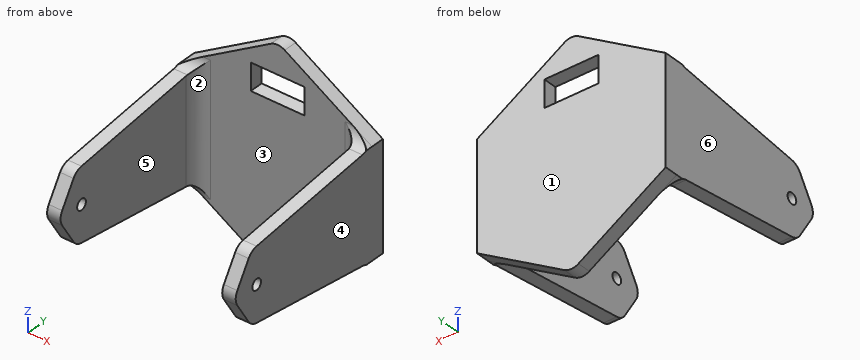
```python
from build123d import *

# Parameters (mm, degrees)
F0_W         = 5
F0_H         = 40
F1_DEPTH     = 70
F3_DEPTH     = 5
F4_R         = 2
F5_DEPTH     = 97.2
F7_DEPTH     = 83.6
F8_T4_DEPTH  = 65
F8_T10_DEPTH = 65
F8_T16_DEPTH = 5
F8_T21_DEPTH = 5
F8_T26_DEPTH = 5
F8_T31_DEPTH = 5
F8_T37_DEPTH = 16.0458347789
F8_T42_DEPTH = 65
F8_T50_DEPTH = 16.0458347789
F8_T55_DEPTH = 65
F8_T63_DEPTH = 16.0458347789
F8_T68_DEPTH = 65
F8_T76_DEPTH = 65
F8_T81_DEPTH = 16.0458347789
F8_T85_DEPTH = 20.294112478
F9_W         = 20
F9_H         = 10
F10_DEPTH    = 25


# Not quite as in the source:
# - a fillet or chamfer that OpenCascade refuses, or shapes differently, is made with other operations: its cross-section is extruded or revolved along the edge and cut away or added


with BuildPart() as f1:
    # F0 (on Front) → F1 (new body)
    with BuildSketch(Plane.XZ):
        with Locations((-32.5, 0)):
            Rectangle(F0_W, F0_H)
    extrude(amount=F1_DEPTH)



with BuildPart() as f1b:
    # F0 (on Front) → F1, piece 2 (new body)
    with BuildSketch(Plane.XZ):
        with Locations((32.5, 0)):
            Rectangle(F0_W, F0_H)
    extrude(amount=F1_DEPTH)


with BuildPart() as f1_1:
    add(f1.part)

    add(f1b.part)  # F3 merges F1b
    # F2 (on face) → F3 (join)
    with BuildSketch(Plane(origin=(0, 0, 0), x_dir=(-1, 0, 0), z_dir=(0, 1, 0))):
        Polygon((-35, -20), (0, -41.4117574692), (35, -20), (35, 20), (0, 41.4117574692), (-35, 20), align=None)
    extrude(amount=F3_DEPTH)

    # F4 (on face) → F5 (cut)
    with BuildSketch(Plane(origin=(-35, 0, 0), x_dir=(0, -1, 0), z_dir=(-1, 0, 0))):
        with Locations((52.9787652194, 0)):
            Circle(F4_R)
    extrude(amount=-F5_DEPTH, mode=Mode.SUBTRACT)

    # F6 (on face) → F7 (cut)
    with BuildSketch(Plane(origin=(-35, 0, 0), x_dir=(0, -1, 0), z_dir=(-1, 0, 0))):
        with BuildLine():
            Line((98.4306931496, 40.8057309687), (0, 20))
            Line((0, 20), (53.01884554, 13.4261534673))
            ThreePointArc((53.01884554, 13.4261534673), (55.107028482, 12.6702755654), (56.6618948527, 11.084636902))
            Line((56.6618948527, 11.084636902), (61.8706015463, 2.6204867239))
            ThreePointArc((61.8706015463, 2.6204867239), (62.6123097139, 0), (61.8706015463, -2.6204867239))
            Line((61.8706015463, -2.6204867239), (56.6618948527, -11.084636902))
            ThreePointArc((56.6618948527, -11.084636902), (55.107028482, -12.6702755654), (53.01884554, -13.4261534673))
            Line((53.01884554, -13.4261534673), (0, -20))
            Line((0, -20), (98.4306931496, -42.0177839696))
            Line((98.4306931496, -42.0177839696), (98.4306931496, 40.8057309687))
        make_face()
    extrude(amount=-F7_DEPTH, mode=Mode.SUBTRACT)

    # F8: fillet of radius 5 on 8 edges, made by hand


with BuildPart() as f8_tool2:
    # F8_s3 → F8_t4 (new body)
    with BuildSketch(Plane.XY.offset(32.5)):
        with BuildLine():
            ThreePointArc((25, 0), (28.5355339059, -1.4644660941), (30, -5))
            Line((30, -5), (30, 0))
            Line((30, 0), (25, 0))
        make_face()
    extrude(amount=-F8_T4_DEPTH)

    split(bisect_by=Plane(origin=(0, -2.4422683248, 19.6971813136), x_dir=(1, 0, 0), z_dir=(0, 0.1230485039, -0.9924006578)), keep=Keep.TOP)

    split(bisect_by=Plane(origin=(0, -2.4422683248, -19.6971813136), x_dir=(1, 0, 0), z_dir=(0, 0.1230485039, 0.9924006578)), keep=Keep.TOP)


with BuildPart() as f1_2:
    add(f1_1.part)

    # F8_t1: union F8_tool2
    add(f8_tool2.part)


with BuildPart() as f8_tool8:
    # F8_s9 → F8_t10 (new body)
    with BuildSketch(Plane.XY.offset(-32.5)):
        with BuildLine():
            ThreePointArc((-25, 0), (-28.5355339059, -1.4644660941), (-30, -5))
            Line((-30, -5), (-30, 0))
            Line((-30, 0), (-25, 0))
        make_face()
    extrude(amount=F8_T10_DEPTH)

    split(bisect_by=Plane(origin=(0, -2.4422683248, -19.6971813136), x_dir=(1, 0, 0), z_dir=(0, 0.1230485039, 0.9924006578)), keep=Keep.TOP)

    split(bisect_by=Plane(origin=(0, -2.4422683248, 19.6971813136), x_dir=(1, 0, 0), z_dir=(0, 0.1230485039, -0.9924006578)), keep=Keep.TOP)


with BuildPart() as f1_3:
    add(f1_2.part)

    # F8_t7: union F8_tool8
    add(f8_tool8.part)


with BuildPart() as f8_tool14:
    # F8_s15 → F8_t16 (new body)
    with BuildSketch(Plane.YZ.offset(35)):
        with BuildLine():
            ThreePointArc((-4.3847574804, 19.4563306223), (-1.2532539052, 21.1074588458), (0, 24.4183339115))
            Line((0, 24.4183339115), (0, 20))
            Line((0, 20), (-4.3847574804, 19.4563306223))
        make_face()
    extrude(amount=-F8_T16_DEPTH)

    split(bisect_by=Plane(origin=(18.4348816442, 0, 30.1339513338), x_dir=(0, 1, 0), z_dir=(-0.5218557601, 0, -0.8530337424)), keep=Keep.TOP)


with BuildPart() as f1_4:
    add(f1_3.part)

    # F8_t13: union F8_tool14
    add(f8_tool14.part)


with BuildPart() as f8_tool19:
    # F8_s20 → F8_t21 (new body)
    with BuildSketch(Plane.YZ.offset(-30)):
        with BuildLine():
            ThreePointArc((0, 24.4183339115), (-1.2532539052, 21.1074588458), (-4.3847574804, 19.4563306223))
            Line((-4.3847574804, 19.4563306223), (0, 20))
            Line((0, 20), (0, 24.4183339115))
        make_face()
    extrude(amount=-F8_T21_DEPTH)

    split(bisect_by=Plane(origin=(-18.4348816442, 0, 30.1339513338), x_dir=(0, 1, 0), z_dir=(0.5218557601, 0, -0.8530337424)), keep=Keep.TOP)


with BuildPart() as f1_5:
    add(f1_4.part)

    # F8_t18: union F8_tool19
    add(f8_tool19.part)


with BuildPart() as f8_tool24:
    # F8_s25 → F8_t26 (new body)
    with BuildSketch(Plane.YZ.offset(-35)):
        with BuildLine():
            ThreePointArc((0, -24.4183339115), (-1.2532539052, -21.1074588458), (-4.3847574804, -19.4563306223))
            Line((-4.3847574804, -19.4563306223), (0, -20))
            Line((0, -20), (0, -24.4183339115))
        make_face()
    extrude(amount=F8_T26_DEPTH)

    split(bisect_by=Plane(origin=(-18.4348816442, 0, -30.1339513338), x_dir=(0, 1, 0), z_dir=(0.5218557601, 0, 0.8530337424)), keep=Keep.TOP)


with BuildPart() as f1_6:
    add(f1_5.part)

    # F8_t23: union F8_tool24
    add(f8_tool24.part)


with BuildPart() as f8_tool29:
    # F8_s30 → F8_t31 (new body)
    with BuildSketch(Plane.YZ.offset(30)):
        with BuildLine():
            ThreePointArc((-4.3847574804, -19.4563306223), (-1.2532539052, -21.1074588458), (0, -24.4183339115))
            Line((0, -24.4183339115), (0, -20))
            Line((0, -20), (-4.3847574804, -19.4563306223))
        make_face()
    extrude(amount=F8_T31_DEPTH)

    split(bisect_by=Plane(origin=(18.4348816442, 0, -30.1339513338), x_dir=(0, 1, 0), z_dir=(-0.5218557601, 0, 0.8530337424)), keep=Keep.TOP)


with BuildPart() as f1_7:
    add(f1_6.part)

    # F8_t28: union F8_tool29
    add(f8_tool29.part)


with BuildPart() as f8_tool35:
    # F8_s36 → F8_t37 (new body)
    with BuildSketch(Plane.YZ.offset(35)):
        with BuildLine():
            ThreePointArc((-4.3847574804, 19.4563306223), (-1.2532539052, 21.1074588458), (0, 24.4183339115))
            Line((0, 24.4183339115), (0, 20))
            Line((0, 20), (-4.3847574804, 19.4563306223))
        make_face()
    extrude(amount=-F8_T37_DEPTH)

    split(bisect_by=Plane(origin=(18.4348816442, 0, 30.1339513338), x_dir=(0, 1, 0), z_dir=(-0.5218557601, 0, -0.8530337424)), keep=Keep.TOP)

    split(bisect_by=Plane.YZ.offset(30), keep=Keep.BOTTOM)


with BuildPart() as f8_tool40:
    # F8_s41 → F8_t42 (new body)
    with BuildSketch(Plane.XY.offset(32.5)):
        with BuildLine():
            ThreePointArc((25, 0), (28.5355339059, -1.4644660941), (30, -5))
            Line((30, -5), (30, 0))
            Line((30, 0), (25, 0))
        make_face()
    extrude(amount=-F8_T42_DEPTH)

    split(bisect_by=Plane(origin=(18.4348816442, 0, 30.1339513338), x_dir=(0, 1, 0), z_dir=(-0.5218557601, 0, -0.8530337424)), keep=Keep.TOP)

    split(bisect_by=Plane(origin=(0, -2.4422683248, 19.6971813136), x_dir=(1, 0, 0), z_dir=(0, -0.1230485039, 0.9924006578)), keep=Keep.TOP)


with BuildPart() as f8_tool35_1:
    add(f8_tool35.part)

    # F8_t45: intersect F8_tool40
    add(f8_tool40.part, mode=Mode.INTERSECT)


with BuildPart() as f1_8:
    add(f1_7.part)

    # F8_t33: union F8_tool35
    add(f8_tool35_1.part)


with BuildPart() as f8_tool48:
    # F8_s49 → F8_t50 (new body)
    with BuildSketch(Plane.YZ.offset(18.9541652211)):
        with BuildLine():
            ThreePointArc((-4.3847574804, -19.4563306223), (-1.2532539052, -21.1074588458), (0, -24.4183339115))
            Line((0, -24.4183339115), (0, -20))
            Line((0, -20), (-4.3847574804, -19.4563306223))
        make_face()
    extrude(amount=F8_T50_DEPTH)

    split(bisect_by=Plane(origin=(18.4348816442, 0, -30.1339513338), x_dir=(0, 1, 0), z_dir=(-0.5218557601, 0, 0.8530337424)), keep=Keep.TOP)

    split(bisect_by=Plane.YZ.offset(30), keep=Keep.BOTTOM)


with BuildPart() as f8_tool53:
    # F8_s54 → F8_t55 (new body)
    with BuildSketch(Plane.XY.offset(32.5)):
        with BuildLine():
            ThreePointArc((25, 0), (28.5355339059, -1.4644660941), (30, -5))
            Line((30, -5), (30, 0))
            Line((30, 0), (25, 0))
        make_face()
    extrude(amount=-F8_T55_DEPTH)

    split(bisect_by=Plane(origin=(18.4348816442, 0, -30.1339513338), x_dir=(0, 1, 0), z_dir=(-0.5218557601, 0, 0.8530337424)), keep=Keep.TOP)

    split(bisect_by=Plane(origin=(0, -2.4422683248, -19.6971813136), x_dir=(1, 0, 0), z_dir=(0, -0.1230485039, -0.9924006578)), keep=Keep.TOP)


with BuildPart() as f8_tool48_1:
    add(f8_tool48.part)

    # F8_t58: intersect F8_tool53
    add(f8_tool53.part, mode=Mode.INTERSECT)


with BuildPart() as f1_9:
    add(f1_8.part)

    # F8_t46: union F8_tool48
    add(f8_tool48_1.part)


with BuildPart() as f8_tool61:
    # F8_s62 → F8_t63 (new body)
    with BuildSketch(Plane.YZ.offset(-35)):
        with BuildLine():
            ThreePointArc((0, -24.4183339115), (-1.2532539052, -21.1074588458), (-4.3847574804, -19.4563306223))
            Line((-4.3847574804, -19.4563306223), (0, -20))
            Line((0, -20), (0, -24.4183339115))
        make_face()
    extrude(amount=F8_T63_DEPTH)

    split(bisect_by=Plane(origin=(-18.4348816442, 0, -30.1339513338), x_dir=(0, 1, 0), z_dir=(0.5218557601, 0, 0.8530337424)), keep=Keep.TOP)

    split(bisect_by=Plane.YZ.offset(-30), keep=Keep.TOP)


with BuildPart() as f8_tool66:
    # F8_s67 → F8_t68 (new body)
    with BuildSketch(Plane.XY.offset(-32.5)):
        with BuildLine():
            ThreePointArc((-25, 0), (-28.5355339059, -1.4644660941), (-30, -5))
            Line((-30, -5), (-30, 0))
            Line((-30, 0), (-25, 0))
        make_face()
    extrude(amount=F8_T68_DEPTH)

    split(bisect_by=Plane(origin=(-18.4348816442, 0, -30.1339513338), x_dir=(0, 1, 0), z_dir=(0.5218557601, 0, 0.8530337424)), keep=Keep.TOP)

    split(bisect_by=Plane(origin=(0, -2.4422683248, -19.6971813136), x_dir=(1, 0, 0), z_dir=(0, -0.1230485039, -0.9924006578)), keep=Keep.TOP)


with BuildPart() as f8_tool61_1:
    add(f8_tool61.part)

    # F8_t71: intersect F8_tool66
    add(f8_tool66.part, mode=Mode.INTERSECT)


with BuildPart() as f1_10:
    add(f1_9.part)

    # F8_t59: union F8_tool61
    add(f8_tool61_1.part)


with BuildPart() as f8_tool74:
    # F8_s75 → F8_t76 (new body)
    with BuildSketch(Plane.XY.offset(-32.5)):
        with BuildLine():
            ThreePointArc((-25, 0), (-28.5355339059, -1.4644660941), (-30, -5))
            Line((-30, -5), (-30, 0))
            Line((-30, 0), (-25, 0))
        make_face()
    extrude(amount=F8_T76_DEPTH)

    split(bisect_by=Plane(origin=(-18.4348816442, 0, 30.1339513338), x_dir=(0, 1, 0), z_dir=(0.5218557601, 0, -0.8530337424)), keep=Keep.TOP)

    split(bisect_by=Plane(origin=(0, -2.4422683248, 19.6971813136), x_dir=(1, 0, 0), z_dir=(0, -0.1230485039, 0.9924006578)), keep=Keep.TOP)


with BuildPart() as f8_tool79:
    # F8_s80 → F8_t81 (new body)
    with BuildSketch(Plane.YZ.offset(-18.9541652211)):
        with BuildLine():
            ThreePointArc((0, 24.4183339115), (-1.2532539052, 21.1074588458), (-4.3847574804, 19.4563306223))
            Line((-4.3847574804, 19.4563306223), (0, 20))
            Line((0, 20), (0, 24.4183339115))
        make_face()
    extrude(amount=-F8_T81_DEPTH)

    split(bisect_by=Plane(origin=(-18.4348816442, 0, 30.1339513338), x_dir=(0, 1, 0), z_dir=(0.5218557601, 0, -0.8530337424)), keep=Keep.TOP)

    split(bisect_by=Plane.YZ.offset(-30), keep=Keep.TOP)


with BuildPart() as f8_tool74_1:
    add(f8_tool74.part)

    # F8_t84: intersect F8_tool79
    add(f8_tool79.part, mode=Mode.INTERSECT)


with BuildPart() as f1_11:
    add(f1_10.part)

    # F8_t72: union F8_tool74
    add(f8_tool74_1.part)

    # F8_s86 → F8_t85 (cut)
    with BuildSketch(Plane.XZ.offset(-12.647056239)):
        with BuildLine():
            ThreePointArc((-2.6092788007, 39.8154933306), (0, 40.5503246188), (2.6092788007, 39.8154933306))
            Line((2.6092788007, 39.8154933306), (0, 41.4117574692))
            Line((0, 41.4117574692), (-2.6092788007, 39.8154933306))
        make_face()
        with BuildLine():
            ThreePointArc((-2.6092788007, -39.8154933306), (0, -40.5503246188), (2.6092788007, -39.8154933306))
            Line((2.6092788007, -39.8154933306), (0, -41.4117574692))
            Line((0, -41.4117574692), (-2.6092788007, -39.8154933306))
        make_face()
    extrude(amount=F8_T85_DEPTH, mode=Mode.SUBTRACT)

    # F9 (on face) → F10 (cut)
    with BuildSketch(Plane.XZ):
        with Locations((0, 25.0998503715)):
            Rectangle(F9_W, F9_H)
    extrude(amount=-F10_DEPTH, mode=Mode.SUBTRACT)


solid = f1_11.part
```
Here's how the part is built. I have some questions about the finished solid (model axes, mm). Face numbers are marked on the shaded views. A direction names the side the tool comes from. Round coordinates to 2 decimals unless told otherwise and drop trailing zeros. Write each loop counter-clockwise with the first axis right and the second up, starting at its lowest first coordinate (ties: lowest second). Pieces come first, ordered by that corner, then holes.
Q1. If we section it at B-B on x = -4.5: Write out the boundary of the cut face in (y, z), plus the area to 3 significant figures.
Q2. Which directions (+Z, -Z, +X, -X, +Y, -Y) give clear straight access to the entire face, cutting with the end or side of a thin tool? Please do the marked faces 5 and 6.
Q3. Please list where these lines run through material, in increasing order: probe 1 along X at (y, z) = (-39.5, 0); probe 2 along Y at (x, z) = (-14, 2.5); probe 3 along X at (y, z) = (-2.5, 13).
Q4. If we section it at A-A on z = 0: Write out the boundary of the cut face in (x, y).
Q5. If we mould it in two halves opening along X, with no side actions, what happens to the marked faces 1, 2, 3 and 4? For each: +X half, -X half, draft (parallel to the pull), parting line (faces both ways), or undercut.
Q6. If we section it at C-C on y = -36.5: Write out the boundary of the cut face in (x, z).
Q7. Will these pins go through, and if not, where does the flat tip stop? P1, Ø2.5, axis at x = -1.5, y = 3.5, coming from the -Z side; P2, Ø3, axis at x = -1, z = -14.5, coming from the -Y side; P3, Ø3.5, axis at y = -52.98, z = 0, coming from the -X side; P4, Ø4, axis at y = 2.5, z = 24.5, coming from the +X side.
Answer below:
1. outline: (0, -38.66) - (5, -38.66) - (5, 20.1) - (0, 20.1) - close; (0, 30.1) - (5, 30.1) - (5, 38.66) - (0, 38.66) - close
1. area: 337 mm2
2. face 5: +Z, -Z, -Y
2. face 6: +Z, -Z, -X, +Y, -Y
3. probe 1: x = -35 to -30, 30 to 35
3. probe 2: y = 0 to 5
3. probe 3: x = -35 to -29.33, 29.33 to 35
4. outline: (-35, -62.61) - (-30, -62.61) - (-30, -54.98) - (-35, -54.98) - close; (-35, -50.98) - (-30, -50.98) - (-30, -5) arc R5 cw to (-25, 0) - (25, 0) arc R5 cw to (30, -5) - (30, -50.98) - (35, -50.98) - (35, 5) - (-35, 5) - close; (30, -62.61) - (35, -62.61) - (35, -54.98) - (30, -54.98) - close
5. face 1: draft
5. face 2: undercut
5. face 3: undercut
5. face 4: +X half
6. outline: (-35, -15.47) - (-30, -15.47) - (-30, 15.47) - (-35, 15.47) - close; (30, -15.47) - (35, -15.47) - (35, 15.47) - (30, 15.47) - close
7. P1: stops at z = -40.54
7. P2: stops at y = 0
7. P3: passes through
7. P4: stops at x = 30.91
